Part model, mm, in its own coordinate system. Face numbers are marked on the shaded views. A direction names the side the tool comes from. Round coordinates to 2 decimals unless told otherwise and drop trailing zeros. Write each loop counter-clockwise with the first axis right and the second up, starting at its lowest first coordinate (ties: lowest second). Pieces come first, ordered by that corner, then holes.
1) Flat gauge pins, fed straight in: pin 1 (4 mm diameter, centred on x = 20, y = 73, fed in from +Z); pin 2 (2 mm diameter, centred on y = 62.5, z = 29, fed in from +X); pin 3 (10 mm diameter, centred on x = 8.5, z = 99, fed in from +Y); pin 4 (12 mm diameter, centred on x = -85, z = 15, fed in from -Y). Where does each tip first touch, or does it go through?
2) Saw through at C-C on y = 140.5. Write the cut outline in (x, z), and give its area (3 significant figures).
3) Drill centre lines: L1, parallel to X at y = 136, z = -45.5; L2, parallel to Y at x = 78, z = -13; L3, parallel to X at y = 23.5, z = -100. Where is each one in solid material? Low to high.
4) Which spindle directions (+Z, -Z, +X, -X, +Y, -Y) get a long thin tool onto all of the face, cutting with end or side? Do the marked faces 5 and 6. Say none if no direction does.
5) Saw through at B-B on z = 0. Write the cut outline in (x, y).
6) Pull direction X, two halves, no side cores. Call the marked faces 1, 2, 3 and 4: +X half, -X half, draft (parallel to the pull), parting line (faces both ways), or undercut.
7) Saw through at A-A on y = 80. Write the cut outline in (x, z).
8) Saw through at D-D on x = 0. Write the cut outline in (y, z).
Autodesk Inventor part; units mm, degrees
ref_plane "YZ Plane" through (0, 0, 0) normal (1, 0, 0) x (0, 1, 0)
ref_plane "XZ Plane" through (0, 0, 0) normal (0, 1, 0) x (-1, 0, 0)
ref_plane "XY Plane" through (0, 0, 0) normal (0, 0, 1) x (1, 0, 0)
sketch "Sketch1" plane through (0, 0, 0) normal (0, 1, 0) x (-1, 0, 0)
  circle A0 centre (0, 0) radius 127
  dimension "swivelBaseDiameter" = 254
extrude "Extrusion1" add sketch "Sketch1" along normal blind 25.4
sketch "Sketch2" plane through (0, 25.4, 0) normal (0, 1, 0) x (1, 0, 0)
  circle A0 centre (0, 0) radius 127 construction
  line L0 (0, -127) -> (0, 127) construction
  line L1 (-25.4, 63.5) -> (-12.7, 63.5)
  line L2 (-12.7, 63.5) -> (-12.7, -63.5)
  line L3 (-12.7, -63.5) -> (-25.4, -63.5)
  line L4 (-25.4, -63.5) -> (-25.4, 63.5)
  line L5 (-127, 0) -> (127, 0) construction
  line L6 (25.4, 63.5) -> (12.7, 63.5)
  line L7 (12.7, 63.5) -> (12.7, -63.5)
  line L8 (12.7, -63.5) -> (25.4, -63.5)
  line L9 (25.4, -63.5) -> (25.4, 63.5)
  point P0 (-12.7, 0)
  point P1 (12.7, 0)
  dimension "armConnectorSeparation" = 12.7
  dimension "armConnectorsThickness" = 12.7
  dimension "armConnectorsSize" = 127
extrude "Extrusion2" add sketch "Sketch2" along normal blind 25.4
sketch "Sketch3" plane through (25.4, 25.4, 63.5) normal (1, 0, 0) x (0, 0, -1)
  circle A0 centre (63.5, 88.9) radius 63.5 construction
  line L0 (127, 25.4) -> (127, 88.9)
  line L1 (0, 25.4) -> (0, 88.9)
  arc A1 (127, 88.9) -> (0, 88.9) centre (63.5, 88.9) ccw
  line L2 (0, 25.4) -> (127, 25.4)
  point P0 (63.5, 25.4)
  dimension "d9" = 127
extrude "Extrusion3" add sketch "Sketch3" against normal up to surface (12.7 mm away)
extrude "Extrusion4" add sketch "Sketch3" against normal up to surface (12.7 mm away) from surface at -38.1
equation "\"armConnectorSeparation\" = 0.5 * armThickness"
equation "\"armConnectorsSize\" = majorDiameter"
equation "\"d9\" = armConnectorsSize"
equation "\"d10\" = armConnectorsSize"
properties part number "Base-Arm Connector"
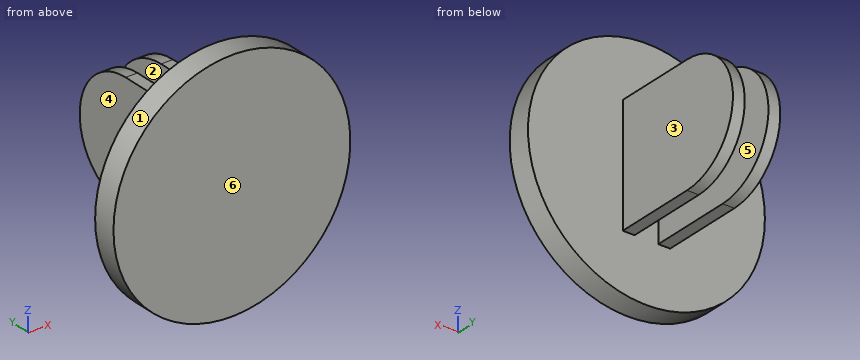
Completed:
1. pin 1: stops at z = 63.5
1. pin 2: stops at x = 25.4
1. pin 3: stops at y = 25.4
1. pin 4: stops at y = 0
2. outline: (-25.4, -57.84) - (-12.7, -57.84) - (-12.7, 57.84) - (-25.4, 57.84) - close; (12.7, -57.84) - (25.4, -57.84) - (25.4, 57.84) - (12.7, 57.84) - close
2. area: 2,940 mm2
3. L1: x = -25.4 to -12.7, 12.7 to 25.4
3. L2: y = 0 to 25.4
3. L3: x = -78.29 to 78.29
4. face 5: +Z, -Z, +Y
4. face 6: +Z, -Z, +X, -X, -Y
5. outline: (-127, 0) - (127, 0) - (127, 25.4) - (25.4, 25.4) - (25.4, 177.8) - (12.7, 177.8) - (12.7, 25.4) - (-12.7, 25.4) - (-12.7, 177.8) - (-25.4, 177.8) - (-25.4, 25.4) - (-127, 25.4) - close
6. face 1: parting line
6. face 2: undercut
6. face 3: +X half
6. face 4: -X half
7. outline: (-25.4, -63.5) - (-12.7, -63.5) - (-12.7, 63.5) - (-25.4, 63.5) - close; (12.7, -63.5) - (25.4, -63.5) - (25.4, 63.5) - (12.7, 63.5) - close
8. outline: (0, -127) - (25.4, -127) - (25.4, 127) - (0, 127) - close
